Model file for the job. Use its own axes, mm. Give positions to 0.01 mm unless a question says otherwise; leave off trailing zeros. Loops run counter-clockwise (first coordinate to the right, second up) from the corner with the lowest first, then second, coordinate; pieces in that order, holes last. Notation, with made-up numbers: (16, -38) - (57, -38) arc R14 ccw to (57, -18) - close; hole circle Ø5 at (-4, 84). An arc over 180 degrees is marked (long way). Use a Markdown table: item, result.
from build123d import *

# Parameters (mm, degrees)
BOSS_EXTRUDE1_DEPTH     = 5
CHAMFER1_SIZE           = 40
SKETCH4_R               = 1.5
CUT_EXTRUDE1_DEPTH      = 10
SKETCH10_R              = 2.25
CUT_EXTRUDE3_DEPTH      = 5
CRVPATTERN1_START       = -46.188021535
CRVPATTERN1_OUTLINE_R   = 2.25
CRVPATTERN1_DEPTH       = 5
CRVPATTERN1_START_2     = -41.188021535
CRVPATTERN1_2_OUTLINE_R = 1.5
CRVPATTERN1_2_DEPTH     = 5
CRVPATTERN1_3_OUTLINE_R = 2.25
CRVPATTERN1_3_DEPTH     = 5
CRVPATTERN1_4_OUTLINE_R = 1.5
CRVPATTERN1_4_DEPTH     = 5
F_3_0MM_DOWEL_HOLE1_D   = 3
SKETCH9_R               = 2.25
CUT_EXTRUDE2_DEPTH      = 5
FILLET1_R               = 3


# Read off the part's stored shape, not the designer's step: CrvPattern1
with BuildPart() as part:
    # Sketch2 → Boss-Extrude1 (new, symmetric)
    with BuildSketch(Plane(origin=(0, 0, 0), x_dir=(1, 0, 0), z_dir=(0, 1, 0))):
        Polygon((70, -40.414518843), (0, 80.829037687), (-70, -40.414518843), align=None)
    extrude(amount=BOSS_EXTRUDE1_DEPTH, both=True)

    # Chamfer1
    chamfer1_edges = [part.edges().sort_by_distance(p)[0] for p in [
        (-70, 0, 40.414518843),
        (0, 0, -80.829037687),
        (70, 0, 40.414518843),
    ]]
    chamfer(chamfer1_edges, length=CHAMFER1_SIZE)

    # Sketch4 → Cut-Extrude1 (cut)
    with BuildSketch(Plane(origin=(40, 0, 23.094010768), x_dir=(0.5000000000000004, 0, -0.8660254037844384), z_dir=(0.8660254037844384, 0, 0.5000000000000004))):
        with Locations((-11, -1)):
            Circle(SKETCH4_R)
        with Locations((11, -1)):
            Circle(SKETCH4_R)
    extrude(amount=-CUT_EXTRUDE1_DEPTH, mode=Mode.SUBTRACT)

    # Sketch10 → Cut-Extrude3 (cut)
    with BuildSketch(Plane(origin=(40, 0, 23.094010768), x_dir=(0.4999999999999997, 0, -0.8660254037844388), z_dir=(0.8660254037844389, 0, 0.49999999999999983))):
        with Locations((-11, -1)):
            Circle(SKETCH10_R)
        with Locations((11, -1)):
            Circle(SKETCH10_R)
    extrude(amount=-CUT_EXTRUDE3_DEPTH, mode=Mode.SUBTRACT)

    # CrvPattern1 outline → CrvPattern1 (cut)
    with BuildSketch(Plane.XY.offset(CRVPATTERN1_START)):
        with Locations((11, -1)):
            Circle(CRVPATTERN1_OUTLINE_R)
        with Locations((-11, -1)):
            Circle(CRVPATTERN1_OUTLINE_R)
    extrude(amount=CRVPATTERN1_DEPTH, mode=Mode.SUBTRACT)

    # CrvPattern1 2 outline → CrvPattern1 2 (cut)
    with BuildSketch(Plane.XY.offset(CRVPATTERN1_START_2)):
        with Locations((11, -1)):
            Circle(CRVPATTERN1_2_OUTLINE_R)
        with Locations((-11, -1)):
            Circle(CRVPATTERN1_2_OUTLINE_R)
    extrude(amount=CRVPATTERN1_2_DEPTH, mode=Mode.SUBTRACT)

    # CrvPattern1 3 outline → CrvPattern1 3 (cut)
    with BuildSketch(Plane(origin=(0, 0, 0), x_dir=(0.500000000000013, 0, 0.8660254037844313), z_dir=(0.8660254037844312, 0, -0.5000000000000131)).offset(CRVPATTERN1_START)):
        with Locations((-11, 1)):
            Circle(CRVPATTERN1_3_OUTLINE_R)
        with Locations((11, 1)):
            Circle(CRVPATTERN1_3_OUTLINE_R)
    extrude(amount=CRVPATTERN1_3_DEPTH, mode=Mode.SUBTRACT)

    # CrvPattern1 4 outline → CrvPattern1 4 (cut)
    with BuildSketch(Plane(origin=(0, 0, 0), x_dir=(0.500000000000013, 0, 0.8660254037844313), z_dir=(0.8660254037844312, 0, -0.5000000000000131)).offset(CRVPATTERN1_START_2)):
        with Locations((-11, 1)):
            Circle(CRVPATTERN1_4_OUTLINE_R)
        with Locations((11, 1)):
            Circle(CRVPATTERN1_4_OUTLINE_R)
    extrude(amount=CRVPATTERN1_4_DEPTH, mode=Mode.SUBTRACT)

    # Ø3.0mm Dowel Hole1 (through all)
    with Locations(Plane(origin=(0, 5, 0), x_dir=(1, 0, 0), z_dir=(0, 1, 0))):
        with Locations((-20, 15), (20, 15), (20, -15), (-20, -15)):
            Hole(F_3_0MM_DOWEL_HOLE1_D / 2)

    # Sketch9 → Cut-Extrude2 (cut)
    with BuildSketch(Plane(origin=(0, 5, 0), x_dir=(1, 0, 0), z_dir=(0, 1, 0))):
        with Locations(Location((-20, 15, 0), (0, 0, 270))):
            Circle(SKETCH9_R)
        with Locations(Location((20, 15, 0), (0, 0, 270))):
            Circle(SKETCH9_R)
        with Locations(Location((20, -15, 0), (0, 0, 270))):
            Circle(SKETCH9_R)
        with Locations(Location((-20, -15, 0), (0, 0, 270))):
            Circle(SKETCH9_R)
    extrude(amount=-CUT_EXTRUDE2_DEPTH, mode=Mode.SUBTRACT)

    # Fillet1
    fillet1_edges = [part.edges().sort_by_distance(p)[0] for p in [
        (20, 0, -46.188021535),
        (50, 0, 5.773502692),
        (-30, 0, 40.414518843),
        (30, 0, 40.414518843),
        (-50, 0, 5.773502692),
        (-20, 0, -46.188021535),
    ]]
    fillet(fillet1_edges, radius=FILLET1_R)


solid = part.part
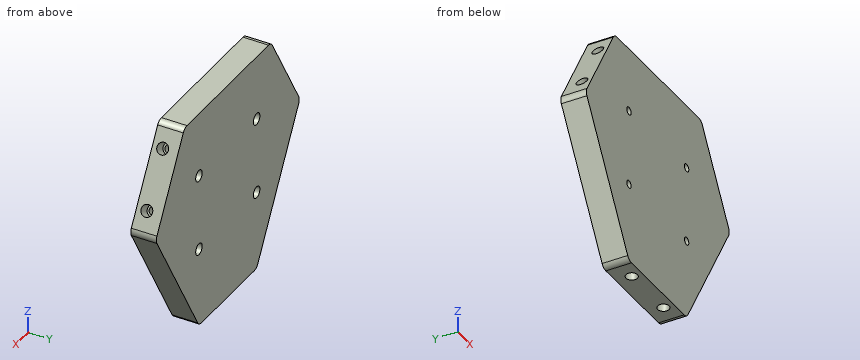
(1) Drill centre lines: probe 1 along Y at (x, z) = (11, -42.45); probe 2 along X at (y, z) = (3.5, -13); probe 3 along Z at (x, y) = (20, -3). Where is each one in solid material? Low to high. Write a range as [from, to].
Computed:
| item | result |
|---|---|
| probe 1 | [-5, -3.25], [1.25, 5] |
| probe 2 | [-39.16, -21.03], [-18.97, 18.97], [21.03, 39.16] |
| probe 3 | [-45.64, -16.5], [-13.5, 13.5], [16.5, 40.41] |
(2) Slice it at B-B, the plane z = -21. Write the cut outline in (x, y).
Computed:
| item | result |
|---|---|
| outline | (-34.54, -5) - (34.54, -5) - (34.54, 5) - (-34.54, 5) - close |
(3) Slice it at A-A, the plane y = 3.75. Write the cut outline in (x, z), plus the area to 3 significant figures.
Computed:
| item | result |
|---|---|
| outline | (-49.13, 4.27) - (-20.87, -44.69) arc R3 ccw to (-18.27, -46.19) - (18.27, -46.19) arc R3 ccw to (20.87, -44.69) - (49.13, 4.27) arc R3 ccw to (49.13, 7.27) - (30.87, 38.91) arc R3 ccw to (28.27, 40.41) - (-28.27, 40.41) arc R3 ccw to (-30.87, 38.91) - (-49.13, 7.27) arc R3 ccw to start; hole circle Ø4.5 at (-20, -15); hole circle Ø4.5 at (-20, 15); hole circle Ø4.5 at (20, -15); hole circle Ø4.5 at (20, 15) |
| area | 6,340 mm² |
(4) Pin check, flat tips, straight feed: P1, Ø1, axis at y = -1.5, z = -30.5, coming from the +X side; P2, Ø0.9, axis at x = 11, y = -1.5, coming from the -Z side; P3, Ø3.5, axis at x = 20, z = 15, coming from the +Y side; P4, Ø2.5, axis at x = 20, z = -15, coming from the +Y side. Stop position of each tip, or through.
Computed:
| item | result |
|---|---|
| P1 | x = 29.35 |
| P2 | z = -36.19 |
| P3 | y = 0 |
| P4 | through |
(5) Slice it at C-C, the plane z = -1.5. Write the cut outline in (x, y).
Computed:
| item | result |
|---|---|
| outline | (-45.8, -5) - (45.8, -5) - (45.8, 5) - (-45.8, 5) - close |
